The model under review builds one solid part; all positions refer to its coordinate system, in mm. A direction names the side the tool comes from. Coordinates: 2 decimals unless noted, no trailing zeros. Write each loop counter-clockwise with the first axis right and the second up, starting at its lowest first coordinate (ties: lowest second). Pieces come first, ordered by that corner, then holes. Notation, with made-up numbers: (60.25, 68.5) -> (70.25, 68.5) arc R32 cw to (70.25, 104.5) -> close; hole circle Ø10 at (83.25, -25.5). An arc over 180 degrees is marked (long way). Put each result on its own line as item: value. Start each with the question number.
from build123d import *

# Parameters (mm, degrees)
F0_W     = 86.4
F0_H     = 54.6
F1_DEPTH = 8
F2_W     = 86.4
F2_H     = 54.6
F3_DEPTH = 3
F4_W     = 86.4
F4_H     = 54.6
F5_DEPTH = 3
F7_DEPTH = 25


with BuildPart() as f1:
    # F0 (on Top) → F1 (new body)
    with BuildSketch(Plane.XY):
        Polygon((-43.2, -27.3), (-43.2, 27.3), (43.2, 27.3), (43.2, 33.3), (-49.2, 33.3), (-49.2, -33.3), (43.2, -33.3), (43.2, -27.3), align=None)
        Rectangle(F0_W, F0_H)
    extrude(amount=F1_DEPTH)

    # F2 (on face) → F3 (cut)
    with BuildSketch(Plane.XY.offset(8)):
        Rectangle(F2_W, F2_H)
    extrude(amount=-F3_DEPTH, mode=Mode.SUBTRACT)

    # F4 (on face) → F5 (cut)
    with BuildSketch(Plane(origin=(0, 0, 0), x_dir=(1, 0, 0), z_dir=(0, 0, -1))):
        Rectangle(F4_W, F4_H)
    extrude(amount=-F5_DEPTH, mode=Mode.SUBTRACT)

    # F6 (on face) → F7 (cut)
    with BuildSketch(Plane(origin=(0, 0, 0), x_dir=(1, 0, 0), z_dir=(0, 0, -1))):
        Polygon((43.2, 33.3), (19.2, 33.3), (43.2, 9.3), align=None)
    extrude(amount=-F7_DEPTH, mode=Mode.SUBTRACT)


solid = f1.part
1. The part is to be moulded in two halves that separate along Y. For faces 4 (the flat face through (28.4, -24.1, 3.9)), 5 (the flat face through (-1, 27.3, 1)), 6 (the flat face through (-44, 5, 8)), 7 (the flat face through (-1, 0, 3)), say which applies: released by +Y, released by -Y, zero draft, split by the parting line, or undercut.
2. Consider section C-C on x = -33.5. State the section outline as (y, z) points, then the cut area to 3 significant figures.
3. Wall thickness on line 1 (Y direction, x = -13.5, z = 7.25); line 2 (X direction, y = 1, z = 0.5); line 3 (Y direction, x = 37, z = 7.5): over which ranges is each line inside the solid? List them lowest first. Write a range as from..to.
4. Consider section A-A on y = -0.5. State the section outline as (x, z) points, then the cut area to 3 significant figures.
5. Consider section B-B on z = 1.75. State the section outline as (x, y) points, then the cut area to 3 significant figures.
6. Insertion check: P1, Ø2.5, axis at y = 0, z = 7, coming from the +X side; P2, Ø1.5, axis at x = 31.5, z = 4, coming from the -Y side; P3, Ø1, axis at x = 19, y = 20.5, coming from the -Z side. Each pin has a flat end and moves straight along its axis. Give the tip position at first contact, or say it passes through.
7. Tool access review of faces 1 (the flat face through (-1, 0, 5)), 2 (the flat face through (-43.2, 0, 1)), 3 (the flat face through (-49.2, 0, 4)): name each direction out of +Z, -Z, +X, -X, +Y, -Y from which nothing blocks a thin tool from reaching the whole face with its end or side.
Output values:
1. face 4: released by -Y
1. face 5: undercut
1. face 6: zero draft
1. face 7: undercut
2. outline: (-33.3, 0) -> (-27.3, 0) -> (-27.3, 3) -> (27.3, 3) -> (27.3, 0) -> (33.3, 0) -> (33.3, 8) -> (27.3, 8) -> (27.3, 5) -> (-27.3, 5) -> (-27.3, 8) -> (-33.3, 8) -> close
2. area: 205 mm^2
3. line 1: y = -33.3..-27.3, 27.3..33.3
3. line 2: x = -49.2..-43.2
3. line 3: y = 27.3..33.3
4. outline: (-49.2, 0) -> (-43.2, 0) -> (-43.2, 3) -> (43.2, 3) -> (43.2, 5) -> (-43.2, 5) -> (-43.2, 8) -> (-49.2, 8) -> close
4. area: 221 mm^2
5. outline: (-49.2, -33.3) -> (19.2, -33.3) -> (25.2, -27.3) -> (-43.2, -27.3) -> (-43.2, 27.3) -> (43.2, 27.3) -> (43.2, 33.3) -> (-49.2, 33.3) -> close
5. area: 1,310 mm^2
6. P1: stops at x = -43.2
6. P2: stops at y = -21.75
6. P3: stops at z = 3
7. face 1: +Z, +X
7. face 2: -Z, +X
7. face 3: +Z, -Z, -X, +Y, -Y
